```python
from build123d import *

# Parameters (mm, degrees)
CROQUIS1_R              = 15
CROQUIS1_W              = 37.5
CROQUIS1_H              = 15
CROQUIS1_R_2            = 2.05
SALIENTE_EXTRUIR1_DEPTH = 5
CROQUIS1_4_R            = 15
SALIENTE_EXTRUIR2_DEPTH = 10
CROQUIS2_R              = 2.95
CORTAR_EXTRUIR1_DEPTH   = 91.863909227


with BuildPart() as part:
    # Croquis1 → Saliente-Extruir1 (new body)
    with BuildSketch(Plane.XY):
        Polygon((67.5, 60), (-52.5, 60), (-52.5, -60), (67.5, -60), (67.5, -7.5), (30, -7.5), (30, 7.5), (67.5, 7.5), align=None)
        Circle(CROQUIS1_R, mode=Mode.SUBTRACT)
        with Locations((48.75, 0)):
            Rectangle(CROQUIS1_W, CROQUIS1_H)
        with Locations((37.55, 0)):
            Circle(CROQUIS1_R_2, mode=Mode.SUBTRACT)
        with Locations((50.05, 0)):
            Circle(CROQUIS1_R_2, mode=Mode.SUBTRACT)
    extrude(amount=SALIENTE_EXTRUIR1_DEPTH)

    # Croquis1<4> → Saliente-Extruir2 (add)
    with BuildSketch(Plane.XY):
        Polygon((67.5, 60), (-52.5, 60), (-52.5, -60), (67.5, -60), (67.5, -7.5), (30, -7.5), (30, 7.5), (67.5, 7.5), align=None)
        Circle(CROQUIS1_4_R, mode=Mode.SUBTRACT)
    extrude(amount=SALIENTE_EXTRUIR2_DEPTH)

    # Croquis2 → Cortar-Extruir1 (cut, through all)
    with BuildSketch(Plane.XY.offset(10)):
        with Locations((49, 17.5)):
            Circle(CROQUIS2_R)
        with Locations((55.25, 27.5)):
            Circle(CROQUIS2_R)
        with Locations((61.5, 17.5)):
            Circle(CROQUIS2_R)
        with Locations(Location((61.5, -17.5, 0), (0, 0, 180))):
            Circle(CROQUIS2_R)
        with Locations(Location((55.25, -27.5, 0), (0, 0, 180))):
            Circle(CROQUIS2_R)
        with Locations(Location((49, -17.5, 0), (0, 0, 180))):
            Circle(CROQUIS2_R)
        with Locations((-42.5, 0)):
            Circle(CROQUIS2_R)
        with Locations((0, 50)):
            Circle(CROQUIS2_R)
        with Locations(Location((0, -50, 0), (0, 0, 180))):
            Circle(CROQUIS2_R)
        with Locations((-40.25, -27.5)):
            Circle(CROQUIS2_R)
        with Locations((-46.5, -17.5)):
            Circle(CROQUIS2_R)
        with Locations((-34, -17.5)):
            Circle(CROQUIS2_R)
        with Locations(Location((-34, 17.5, 0), (0, 0, 180))):
            Circle(CROQUIS2_R)
        with Locations(Location((-46.5, 17.5, 0), (0, 0, 180))):
            Circle(CROQUIS2_R)
        with Locations(Location((-40.25, 27.5, 0), (0, 0, 180))):
            Circle(CROQUIS2_R)
    extrude(amount=-CORTAR_EXTRUIR1_DEPTH, mode=Mode.SUBTRACT)


solid = part.part
```
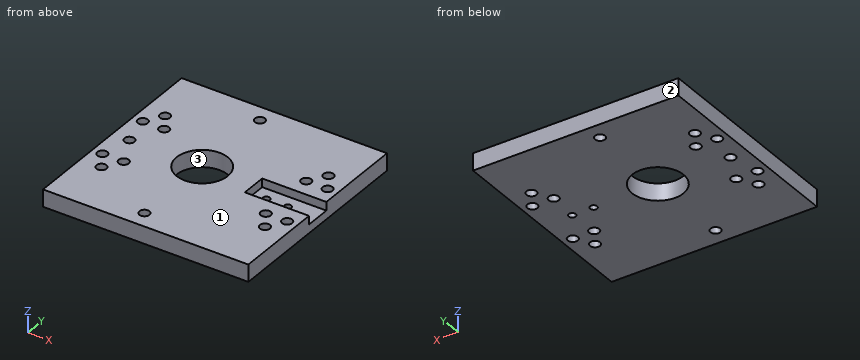
The listing builds one solid part. Answer for the finished solid, in the listing's coordinates (mm). Face numbers are marked on the shaded views. Coordinates: 2 decimals unless noted, no trailing zeros. Write each loop counter-clockwise with the first axis right and the second up, starting at its lowest first coordinate (ties: lowest second). Pieces come first, ordered by that corner, then holes. Notation, with made-up numbers: (-17.75, 3) - (16.25, 3) arc R29 ccw to (16.25, 29) - close; hole circle Ø4 at (59.25, -1). An arc over 180 degrees is marked (long way). Return JSON: item names as keys, results as strings. Group by question number.
1. Determine the mould class of the marked faces 1, 2 and 3 for opening direction Y: released by +Y, released by -Y, zero draft, split by the parting line, or undercut.
2. A cutting plane is placed at B-B, the plane z = 7.75. Give the number of separate pieces and of enclosed holes in the cut face, plus the area to 3 significant figures.
3. A cutting plane is placed at A-A, the plane x = -34. Determine the outline of the cut face in (y, z).
4. Given pin 1 (9.5 mm diameter, centred on x = -46.5, y = -17.5, fed in from +Z); pin 2 (3.5 mm diameter, centred on x = 37.55, y = 0, fed in from +Z); pin 3 (4 mm diameter, centred on y = -1.5, z = 7.5, fed in from +X), each flat-ended and moving along its own axis, determine where each tip first touches the part or whether it passes through.
5. A cutting plane is placed at C-C, the plane y = 27.5. Determine the outline of the cut face in (x, z).
6. A cutting plane is placed at D-D, the plane x = 8. Determine the outline of the cut face in (y, z), plus the area to 3 significant figures.
7. Straight lines are drawn through the part: L1, parallel to Y at x = -34, z = 4; L2, parallel to Y at x = 37.55, z = 2.1; L3, parallel to Y at x = 61.5, z = 7. For each, find the intervals that lie inside material, in ascending order.
Ans:
{
 "1": {"face 1": "zero draft", "face 2": "released by +Y", "face 3": "undercut"},
 "2": {"separate pieces": "1", "enclosed holes": "16", "area": "12,700 mm²"},
 "3": {"outline": "(-60, 0) - (-20.45, 0) - (-20.45, 10) - (-60, 10) - close; (-14.55, 0) - (14.55, 0) - (14.55, 10) - (-14.55, 10) - close; (20.45, 0) - (60, 0) - (60, 10) - (20.45, 10) - close"},
 "4": {"pin 1": "z = 10", "pin 2": "through", "pin 3": "x = 30"},
 "5": {"outline": "(-52.5, 0) - (-43.2, 0) - (-43.2, 10) - (-52.5, 10) - close; (-37.3, 0) - (52.3, 0) - (52.3, 10) - (-37.3, 10) - close; (58.2, 0) - (67.5, 0) - (67.5, 10) - (58.2, 10) - close"},
 "6": {"outline": "(-60, 0) - (-12.69, 0) - (-12.69, 10) - (-60, 10) - close; (12.69, 0) - (60, 0) - (60, 10) - (12.69, 10) - close", "area": "946 mm²"},
 "7": {"L1": "-60 to -20.45, -14.55 to 14.55, 20.45 to 60", "L2": "-60 to -2.05, 2.05 to 60", "L3": "-60 to -20.45, -14.55 to -7.5, 7.5 to 14.55, 20.45 to 60"}
}
